```python
from build123d import *

# Parameters (mm, degrees)
PAD_DEPTH            = 10
PAD001_DEPTH         = 35
SKETCH002_R          = 11.288681
PAD002_DEPTH         = 35
POCKET_DEPTH         = 35.001
SKETCH007_R          = 5.396652
POCKET001_DEPTH      = 10.001
POCKET001_DEPTH_BACK = -35.001
POCKET002_DEPTH      = 10.001
PAD003_DEPTH         = 6
SKETCH010_R          = 4.396251
POCKET003_DEPTH      = 7
SKETCH011_W          = 103.305298
SKETCH011_H          = 76.018318
POCKET004_DEPTH      = 23.748608
POCKET004_DEPTH_BACK = -29.743303


with BuildPart() as part:
    # Sketch → Pad (new body)
    with BuildSketch(Plane.XY):
        with BuildLine():
            ThreePointArc((-34.005628, 23.747608), (-44.43431, 19.427907), (-48.754011, 8.999225))
            Line((-48.754011, -8.999225), (-48.754011, 8.999225))
            ThreePointArc((-48.754011, -8.999225), (-44.43431, -19.427907), (-34.005628, -23.747608))
            Line((34.005628, -23.747608), (-34.005628, -23.747608))
            ThreePointArc((34.005628, -23.747608), (44.43431, -19.427907), (48.754011, -8.999225))
            Line((48.754011, 8.999225), (48.754011, -8.999225))
            ThreePointArc((48.754011, 8.999225), (44.43431, 19.427907), (34.005628, 23.747608))
            Line((-34.005628, 23.747608), (34.005628, 23.747608))
        make_face()
    extrude(amount=PAD_DEPTH)

    # Sketch001 (on Face10 of Pad) → Pad001 (join)
    with BuildSketch(Plane.XY.offset(10)):
        with BuildLine():
            ThreePointArc((17.546094, -23.742303), (29.522235, 0), (17.546094, 23.742303))
            Line((17.546094, 23.742303), (-17.546094, 23.742303))
            ThreePointArc((-17.546094, 23.742303), (-29.522235, 0), (-17.546094, -23.742303))
            Line((-17.546094, -23.742303), (17.546094, -23.742303))
        make_face()
        with BuildLine():
            ThreePointArc((16.156479, -18.892303), (24.858619, 0), (16.156479, 18.892303))
            Line((-16.156479, 18.892303), (16.156479, 18.892303))
            ThreePointArc((-16.156479, 18.892303), (-24.858619, 0), (-16.156479, -18.892303))
            Line((-16.156479, -18.892303), (16.156479, -18.892303))
        make_face(mode=Mode.SUBTRACT)
    extrude(amount=PAD001_DEPTH)

    # Sketch002 (on Face5 of Pad001) → Pad002 (join)
    with BuildSketch(Plane.XY.offset(10)):
        with Locations((32.303345, 0)):
            Circle(SKETCH002_R)
        with Locations((-32.303345, 0)):
            Circle(SKETCH002_R)
    extrude(amount=PAD002_DEPTH)

    # Sketch004 → Pocket (cut, through all)
    with BuildSketch(Plane.XY.offset(10)):
        with BuildLine():
            ThreePointArc((16.156479, -18.892303), (24.858619, 0), (16.156479, 18.892303))
            Line((-16.156479, 18.892303), (16.156479, 18.892303))
            ThreePointArc((-16.156479, 18.892303), (-24.858619, 0), (-16.156479, -18.892303))
            Line((-16.156479, -18.892303), (16.156479, -18.892303))
        make_face()
    extrude(amount=POCKET_DEPTH, mode=Mode.SUBTRACT)

    # Sketch007 → Pocket001 (cut, two sides)
    with BuildSketch(Plane.XY.offset(10)) as pocket001_sk:
        with Locations((32.303345, 0)):
            Circle(SKETCH007_R)
        with Locations((-32.303345, 0)):
            Circle(SKETCH007_R)
    extrude(amount=-POCKET001_DEPTH, mode=Mode.SUBTRACT)
    extrude(pocket001_sk.sketch, amount=-POCKET001_DEPTH_BACK, mode=Mode.SUBTRACT)

    # Sketch008 (on Face38 of Pocket001) → Pocket002 (cut, through all)
    with BuildSketch(Plane.XY.offset(10)):
        with BuildLine():
            ThreePointArc((-8.403063, -3.686291), (0, -9.176067), (8.403063, -3.686291))
            Line((8.403063, -3.686291), (15.352968, -3.686291))
            Line((15.352968, -3.686291), (15.352968, 3.686291))
            Line((15.352968, 3.686291), (8.403063, 3.686291))
            ThreePointArc((8.403063, 3.686291), (0, 9.176067), (-8.403063, 3.686291))
            Line((-8.403063, 3.686291), (-15.352968, 3.686291))
            Line((-15.352968, 3.686291), (-15.352968, -3.686291))
            Line((-15.352968, -3.686291), (-8.403063, -3.686291))
        make_face()
    extrude(amount=-POCKET002_DEPTH, mode=Mode.SUBTRACT)

    # Sketch009 (on Face29 of Pocket002) → Pad003 (join)
    with BuildSketch(Plane.XZ.offset(23.742303)):
        with BuildLine():
            ThreePointArc((-9.139607, 25.729681), (0, 16.590074), (9.139607, 25.729681))
            Line((9.139607, 25.729681), (9.139607, 62.288109))
            ThreePointArc((9.139607, 62.288109), (0, 71.427716), (-9.139607, 62.288109))
            Line((-9.139607, 62.288109), (-9.139607, 25.729681))
        make_face()
    extrude(amount=PAD003_DEPTH)

    # Sketch010 (on Face29 of Pocket002) → Pocket003 (cut, symmetric)
    with BuildSketch(Plane.XZ.offset(23.742303)):
        with Locations((0, 25.729681)):
            Circle(SKETCH010_R)
    extrude(amount=POCKET003_DEPTH, both=True, mode=Mode.SUBTRACT)

    # Sketch011 → Pocket004 (cut, two sides)
    with BuildSketch(Plane.XZ) as pocket004_sk:
        with Locations((0, 81.785393)):
            Rectangle(SKETCH011_W, SKETCH011_H)
    extrude(amount=-POCKET004_DEPTH, mode=Mode.SUBTRACT)
    extrude(pocket004_sk.sketch, amount=-POCKET004_DEPTH_BACK, mode=Mode.SUBTRACT)


solid = part.part
```
Could you check a few things on this model? Use its own coordinates, in mm. A direction names the side the tool comes from. Give positions to 0.01 mm unless a question says otherwise; leave off trailing zeros. Loops run counter-clockwise (first coordinate to the right, second up) from the corner with the lowest first, then second, coordinate; pieces in that order, holes last. Notation, with made-up numbers: (38, 67) - (65, 67) arc R16 cw to (65, 74) - close; hole circle Ø2 at (12.5, -22). An arc over 180 degrees is marked (long way). Answer in a Markdown table with one row per item. Add a question column.
Q1. If we section it at A-A (z = 31.5): List the corners of the cut face in (x, y) for me, plus the area to 3 significant figures.
Q2. If we section it at B-B (y = 0): List the corners of the cut face in (x, z) for me.
Q3. If we section it at C-C (x = 0): State how many separate pieces and enclosed holes the cut face has, plus the area to 3 significant figures.
Q4. Which directions (+Z, -Z, +X, -X, +Y, -Y) give clear straight access to the entire face, cutting with the end or side of a thin tool? Please do faces 4 (the face through (-0.953, -24.393, 21.438)), 5 (the face through (-0.201, -26.7, 16.592)), 6 (the face through (-9.14, -27, 35)), 7 (the face through (-22, -21, 10)).
Q5. If we section it at D-D (x = 29): List the corners of the cut face in (y, z) for me.
Q6. We'd pull the mould along Y, two halves only. Please class faces 1 (the face through (0, -23.742, 15)), 2 (the face through (-1, -10, 0)), 3 (the face through (-12, 3.686, 5)): +Y half, -Y half, draft (parallel to the pull), parting line (faces both ways), or undercut.
Q7. Please list where these lines run through material, in increasing order: L1, parallel to Z at x = 0, y = -22; L2, parallel to X at y = -0.5, z = 38; L3, parallel to Z at x = 22, y = -20. Write a range as from..to.
Q8. For pin 1 (5 mm diameter, centred on x = -10.5, z = 25.5, fed in from -Y); pin 2 (5 mm diameter, centred on x = 13, y = 3.5, fed in from +Z); pin 3 (5 mm diameter, centred on y = 14, z = 35.5, fed in from +X); pin 4 (2 mm diameter, centred on x = -12.5, z = 6, fed in from -Y), each with a flat end and sliding along its axis, tell me the tip position at first contact or that it passes through.
The answers:
| question | item | result |
|---|---|---|
| 1 | outline | (-27.67, -10.29) arc R29.52 ccw to (-17.55, -23.74) - (-9.14, -23.74) - (-9.14, -29.74) - (9.14, -29.74) - (9.14, -23.74) - (17.55, -23.74) arc R29.52 ccw to (27.67, -10.29) arc R11.29 ccw (long way) to (27.67, 10.29) arc R29.52 ccw to (17.55, 23.74) - (-17.55, 23.74) arc R29.52 ccw to (-27.67, 10.29) arc R11.29 ccw (long way) to start; hole circle Ø10.79 at (-32.3, 0); hole (-16.16, -18.89) - (16.16, -18.89) arc R24.86 ccw to (16.16, 18.89) - (-16.16, 18.89) arc R24.86 ccw to start; hole circle Ø10.79 at (32.3, 0) |
| 1 | area | 1,260 mm^2 |
| 2 | outline | (-48.75, 0) - (-37.7, 0) - (-37.7, 43.78) - (-43.59, 43.78) - (-43.59, 10) - (-48.75, 10) - close; (-26.91, 0) - (-15.35, 0) - (-15.35, 10) - (-24.86, 10) - (-24.86, 43.78) - (-26.91, 43.78) - close; (15.35, 0) - (26.91, 0) - (26.91, 43.78) - (24.86, 43.78) - (24.86, 10) - (15.35, 10) - close; (37.7, 0) - (48.75, 0) - (48.75, 10) - (43.59, 10) - (43.59, 43.78) - (37.7, 43.78) - close |
| 3 | separate pieces | 3 |
| 3 | enclosed holes | 0 |
| 3 | area | 687 mm^2 |
| 4 | face 4 | -Y |
| 4 | face 5 | -Z, -Y |
| 4 | face 6 | +Z, -Z, -X, -Y |
| 4 | face 7 | +Z |
| 5 | outline | (-23.75, 0) - (-4.27, 0) - (-4.27, 43.78) - (-10.79, 43.78) - (-10.79, 10) - (-23.75, 10) - close; (4.27, 0) - (23.75, 0) - (23.75, 10) - (10.79, 10) - (10.79, 43.78) - (4.27, 43.78) - close |
| 6 | face 1 | -Y half |
| 6 | face 2 | draft |
| 6 | face 3 | undercut |
| 7 | L1 | z = 0..21.33, 30.13..43.78 |
| 7 | L2 | x = -43.58..-37.68, -26.93..-24.85, 24.85..26.93, 37.68..43.58 |
| 7 | L3 | z = 0..10 |
| 8 | pin 1 | stops at y = -29.74 |
| 8 | pin 2 | stops at z = 10 |
| 8 | pin 3 | stops at x = 27.19 |
| 8 | pin 4 | stops at y = -23.75 |
